from build123d import *

# Parameters (mm, degrees)
ESBO_O1_R                     = 14
RESSALTO_EXTRUS_O3_DEPTH      = 18
ESBO_O3_R                     = 14
ESBO_O3_R_2                   = 12.5
RESSALTO_EXTRUS_O4_DEPTH      = 6
ESBO_O4_R                     = 4.5
CORTE_EXTRUS_O1_DEPTH         = 47.787712062
FURO_ROSCADO_DE_M3X0_51_D     = 2.5
FURO_ROSCADO_DE_M3X0_51_DEPTH = 7.5
FURO_ROSCADO_DE_M3X0_51_TIP   = 0.751075774


with BuildPart() as part:
    # Esboço1 → Ressalto-extrusão3 (new body)
    with BuildSketch(Plane.XY):
        Polygon((-35, 0), (35, 0), (35, 19.7), (18, 19.7), (18, 38.7), (-18, 38.7), (-18, 19.7), (-35, 19.7), align=None)
        with Locations((0, 20.7)):
            Circle(ESBO_O1_R, mode=Mode.SUBTRACT)
    extrude(amount=RESSALTO_EXTRUS_O3_DEPTH)

    # Esboço3 → Ressalto-extrusão4 (add)
    # profile 1 of 2: a face of its own
    with BuildSketch(Plane.XY.offset(18)):
        Polygon((35, 0), (35, 19.7), (18, 19.7), (18, 38.7), (-18, 38.7), (-18, 19.7), (-35, 19.7), (-35, 0), align=None)
        with Locations((0, 20.7)):
            Circle(ESBO_O3_R, mode=Mode.SUBTRACT)
    # profile 2 of 2: a face of its own
    with BuildSketch(Plane.XY.offset(18)):
        with Locations((0, 20.7)):
            Circle(ESBO_O3_R)
        with Locations((0, 20.7)):
            Circle(ESBO_O3_R_2, mode=Mode.SUBTRACT)
    extrude(amount=RESSALTO_EXTRUS_O4_DEPTH)

    # Esboço4 → Corte-extrusão1 (cut, through all)
    with BuildSketch(Plane(origin=(0, 19.7, 0), x_dir=(1, 0, 0), z_dir=(0, 1, 0))):
        with Locations(Location((-26, -12, 0), (0, 0, 180))):
            Circle(ESBO_O4_R)
        with Locations((26, -12)):
            Circle(ESBO_O4_R)
    extrude(amount=-CORTE_EXTRUS_O1_DEPTH, mode=Mode.SUBTRACT)

    # Furo roscado de M3x0.51
    with Locations(Plane(origin=(0, 0, 0), x_dir=(-1, 0, 0), z_dir=(0, 0, -1))):
        with Locations((14.142135624, 34.842135624), (14.142135624, 6.557864376), (-14.142135624, 6.557864376), (-14.142135624, 34.842135624)):
            Hole(FURO_ROSCADO_DE_M3X0_51_D / 2, depth=FURO_ROSCADO_DE_M3X0_51_DEPTH)
            with Locations((0, 0, -(FURO_ROSCADO_DE_M3X0_51_DEPTH + FURO_ROSCADO_DE_M3X0_51_TIP / 2))):  # 118° drill point
                Cone(0, FURO_ROSCADO_DE_M3X0_51_D / 2, FURO_ROSCADO_DE_M3X0_51_TIP, mode=Mode.SUBTRACT)


solid = part.part
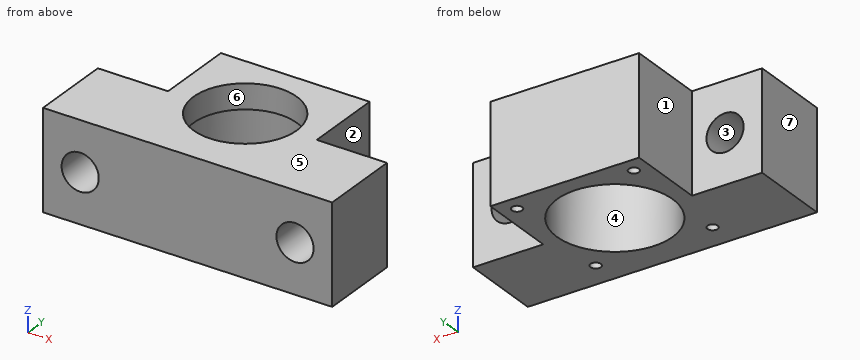
Model file for the job. Use its own axes, mm. Face numbers are marked on the shaded views. A direction names the side the tool comes from. Give positions to 0.01 mm unless a question says otherwise; leave off trailing zeros. Loops run counter-clockwise (first coordinate to the right, second up) from the corner with the lowest first, then second, coordinate; pieces in that order, holes last. Notation, with made-up numbers: (-37, 63.5) - (-26, 63.5) arc R26 ccw to (-26, 78.5) - close; hole circle Ø2 at (-16.75, 10.5). An arc over 180 degrees is marked (long way). Use one line per item in the form item = value.
(1) 3-axis set-ups, long thin cutter, end or side, ignore diameter. For the marked faces 1, 2, 3 and 4: which of +Z, -Z, +X, -X, +Y, -Y reach the whole face in a straight line?
Determined:
face_1 = +Z, -Z, -X, +Y
face_2 = +Z, -Z, +X, +Y
face_3 = +Y, -Y
face_4 = -Z
(2) Cut at B-B (x = -26). Give the cut face in (y, z), then the cut area to 4 significant figures.
Determined:
outline = (0, 0) - (19.7, 0) - (19.7, 7.5) - (0, 7.5) - close; (0, 16.5) - (19.7, 16.5) - (19.7, 24) - (0, 24) - close
area = 295.5 mm^2
(3) Pull direction X, two halves, no side cores. Call the marked faces 5, 6 and 7: pulls with the +X half, pulls with the -X half, needs draft (parallel to the pull), parting line crosses it, or undercut.
Determined:
face_5 = needs draft
face_6 = undercut
face_7 = pulls with the -X half
(4) Drill centre lines: L1, parallel to X at y = 9, z = 10.75; L2, parallel to Y at x = 0, z = 9.75; L3, parallel to X at y = 9.5, z = 14.5. Where is each one in solid material? Low to high.
Determined:
L1 = -35 to -30.32, -21.68 to -7.69, 7.69 to 21.68, 30.32 to 35
L2 = 0 to 6.7, 34.7 to 38.7
L3 = -35 to -29.74, -22.26 to -8.4, 8.4 to 22.26, 29.74 to 35
(5) Cut at C-C (y = 9). Give the cut face in (x, z).
Determined:
outline = (-35, 0) - (-7.69, 0) - (-7.69, 18) - (-4.4, 18) - (-4.4, 24) - (-35, 24) - close; (4.4, 18) - (7.69, 18) - (7.69, 0) - (35, 0) - (35, 24) - (4.4, 24) - close; hole circle Ø9 at (-26, 12); hole circle Ø9 at (26, 12)
(6) Cut at A-A (z = 12). Give the cut face in (x, y).
Determined:
outline = (-35, 0) - (-30.5, 0) - (-30.5, 19.7) - (-35, 19.7) - close; (-21.5, 0) - (21.5, 0) - (21.5, 19.7) - (18, 19.7) - (18, 38.7) - (-18, 38.7) - (-18, 19.7) - (-21.5, 19.7) - close; (30.5, 0) - (35, 0) - (35, 19.7) - (30.5, 19.7) - close; hole circle Ø28 at (0, 20.7)
(7) Drop flat-ended pins along their axis: P1, Ø9.5, axis at y = 25.5, z = 17.5, coming from the +X side; P2, Ø2, axis at x = -14.14, y = 6.56, coming from the -Z side; P3, Ø7, axis at x = -26, z = 12, coming from the +Y side; P4, Ø13.5, axis at x = -25, z = 16.5, coming from the +Y side. Give the stop position or say it passes through.
Determined:
P1 = 18
P2 = 7.65
P3 = through
P4 = 19.7
(8) Cut at D-D (z = 22.75). Give the cut face in (x, y).
Determined:
outline = (-35, 0) - (35, 0) - (35, 19.7) - (18, 19.7) - (18, 38.7) - (-18, 38.7) - (-18, 19.7) - (-35, 19.7) - close; hole circle Ø25 at (0, 20.7)
